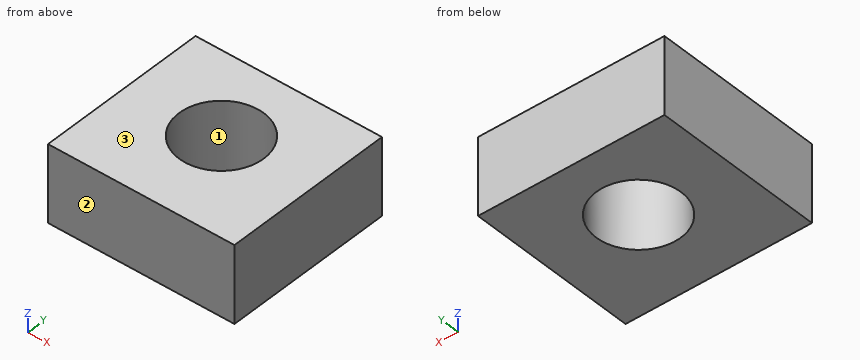
Autodesk Inventor part; units mm, degrees
ref_plane "YZ Plane" through (0, 0, 0) normal (1, 0, 0) x (0, 1, 0)
ref_plane "XZ Plane" through (0, 0, 0) normal (0, 1, 0) x (-1, 0, 0)
ref_plane "XY Plane" through (0, 0, 0) normal (0, 0, 1) x (1, 0, 0)
sketch "Skizze1" plane through (0, 0, 0) normal (0, 0, 1) x (1, 0, 0)
  line L0 (3.75, 4.9488) -> (3.75, -1.9512)
  line L1 (-3.75, -1.9512) -> (-3.75, 4.9488)
  line L2 (3.75, -1.9512) -> (-3.75, -1.9512)
  line L3 (0, 0) -> (3.75, 0) construction
  line L4 (0, 1.7988) -> (0, -1.9512) construction
  line L5 (-3.75, 4.9488) -> (3.75, 4.9488)
  line L6 (3.75, 4.9488) -> (3.75, -1.9512)
  line L7 (3.75, -1.9512) -> (-3.75, -1.9512)
  line L8 (-3.75, -1.9512) -> (-3.75, 4.9488)
  circle A0 centre (0, 1.7988) radius 1.7
  dimension "d0" = 3.75
  dimension "d2" = 3.75
  dimension "d5" = 3.4
extrude "Extrusion2" add sketch "Skizze1" against normal blind 3.1
thread "Gewinde1"
properties part number "mutter"
Verification items for the finished model (mm, model axes). Face numbers are marked on the shaded views. Round coordinates to 2 decimals unless told otherwise and drop trailing zeros. Write each loop counter-clockwise with the first axis right and the second up, starting at its lowest first coordinate (ties: lowest second). Pieces come first, ordered by that corner, then holes.
1. Section check C-C on z = -0.6. Enter the section's corners in (x, y), plus the area to 3 significant figures.
2. Section check B-B on y = 2.75. Enter the section's corners in (x, z).
3. Scan lines: L1, parallel to Y at x = 0, z = -1.1; L2, parallel to Y at x = -1.5, z = -0.9; L3, parallel to X at y = 2.75, z = -1.3. Record each from-to range of solid material in increasing order.
4. Draft check along Y on the marked faces 1, 2 and 3. Enter one of: +Y half, -Y half, draft (parallel to the pull), parting line (faces both ways), or undercut.
5. Section check A-A on x = 0. Enter the section's corners in (y, z), plus the area to 4 significant figures.
Answer:
1. outline: (-3.75, -1.95) - (3.75, -1.95) - (3.75, 4.95) - (-3.75, 4.95) - close; hole circle Ø3.4 at (0, 1.8)
1. area: 42.7 mm2
2. outline: (-3.75, -3.1) - (-1.41, -3.1) - (-1.41, 0) - (-3.75, 0) - close; (1.41, -3.1) - (3.75, -3.1) - (3.75, 0) - (1.41, 0) - close
3. L1: y = -1.95 to 0.1, 3.5 to 4.95
3. L2: y = -1.95 to 1, 2.6 to 4.95
3. L3: x = -3.75 to -1.41, 1.41 to 3.75
4. face 1: undercut
4. face 2: -Y half
4. face 3: draft
5. outline: (-1.95, -3.1) - (0.1, -3.1) - (0.1, 0) - (-1.95, 0) - close; (3.5, -3.1) - (4.95, -3.1) - (4.95, 0) - (3.5, 0) - close
5. area: 10.85 mm2
